from build123d import *

# Parameters (mm, degrees)
SKETCH1_W           = 254
SKETCH1_H           = 58.42
BOSS_EXTRUDE1_DEPTH = 19.05
CUT_EXTRUDE1_DEPTH  = 6.35
FILLET1_R           = 9.525
CUT_EXTRUDE2_START  = -127
SKETCH4_W           = 63.359739346
SKETCH4_H           = 23.579054397
CUT_EXTRUDE2_DEPTH  = 127
SKETCH5_R           = 3.175
CUT_EXTRUDE3_DEPTH  = 15.24
SKETCH6_W           = 12.7
SKETCH6_H           = 21.082
BOSS_EXTRUDE2_DEPTH = 6.35


with BuildPart() as part:
    # Sketch1 → Boss-Extrude1 (new body)
    with BuildSketch(Plane(origin=(0, 0, 0), x_dir=(1, 0, 0), z_dir=(0, 1, 0))):
        with Locations((127, 29.21)):
            Rectangle(SKETCH1_W, SKETCH1_H)
    extrude(amount=BOSS_EXTRUDE1_DEPTH)

    # Sketch2 → Cut-Extrude1 (cut)
    with BuildSketch(Plane(origin=(0, 19.05, 0), x_dir=(1, 0, 0), z_dir=(0, 1, 0))):
        Polygon((221.234, 52.07), (221.234, 18.288), (127, 18.288), (127, 0), (254, 0), (254, 58.42), (127, 58.42), (127, 52.07), align=None)
        Polygon((127, 0), (127, 18.288), (32.766, 18.288), (32.766, 52.07), (127, 52.07), (127, 58.42), (0, 58.42), (0, 0), align=None)
    extrude(amount=-CUT_EXTRUDE1_DEPTH, mode=Mode.SUBTRACT)

    # Fillet1
    fillet1_edges = [part.edges().sort_by_distance(p)[0] for p in [
        (254, 0, -29.21),
        (0, 0, -29.21),
    ]]
    fillet(fillet1_edges, radius=FILLET1_R)

    # Sketch4 → Cut-Extrude2 (cut)
    with BuildSketch(Plane(origin=(254, 0, 0), x_dir=(0, 0, -1), z_dir=(1, 0, 0)).offset(CUT_EXTRUDE2_START)):
        with Locations((31.679869673, 11.789527199)):
            Rectangle(SKETCH4_W, SKETCH4_H)
    extrude(amount=CUT_EXTRUDE2_DEPTH, mode=Mode.SUBTRACT)

    # Sketch5 → Cut-Extrude3 (cut)
    with BuildSketch(Plane(origin=(127, 0, 0), x_dir=(0, 0, -1), z_dir=(1, 0, 0))):
        with Locations((16.51, 6.35)):
            Circle(SKETCH5_R)
        with Locations((29.21, 6.35)):
            Circle(SKETCH5_R)
        with Locations((41.91, 6.35)):
            Circle(SKETCH5_R)
    extrude(amount=-CUT_EXTRUDE3_DEPTH, mode=Mode.SUBTRACT)

    # Sketch6 → Boss-Extrude2 (add)
    with BuildSketch(Plane(origin=(0, 12.7, 0), x_dir=(1, 0, 0), z_dir=(0, 1, 0))):
        with Locations((26.416, 28.829)):
            Rectangle(SKETCH6_W, SKETCH6_H)
    extrude(amount=BOSS_EXTRUDE2_DEPTH)


solid = part.part
Can you work these out from the model? Positions are in its coordinate system, mm. A direction names the side the tool comes from. Give positions to 0.01 mm unless a question says otherwise; leave off trailing zeros. Order: outer loops, then holes, each group sorted by start corner. A loop starts at its lowest first (then second) coordinate and runs counter-clockwise, first axis right, second up. Notation, with made-up numbers: M 88,19.5 L 139,19.5 A19 ccw 139,29.5 Z; hole C 72.25,-6.75 d5. An arc over 180 degrees is marked long. Use one line per item in the form item = value. Start each with the question number.
Item 1: Will these pins go through, and if not, where does the flat tip stop? pin 1 Ø7 at (x, y) = (25, 15.5) entering from -Z; pin 2 Ø4 at (y, z) = (6.35, -29.21) entering from +X; pin 3 Ø2 at (y, z) = (5.5, -6) entering from -X; pin 4 Ø1.5 at (y, z) = (16.5, -49.5) entering from -X.
Item 2: If we section it at B-B (x = 114): Write out the boundary of the cut face in (y, z) (3 decimals).
Item 3: We'd pull the mould along Y, two halves only. Please class faces 1 (the flat face through (73, 16, -18.288)), 2 (the flat face through (73, 19.05, -35)), 3 (the flat face through (111.76, 6, -42)), 4 (the cylindrical face through (2.72, 2.86, -29.62)): +Y half, -Y half, draft (parallel to the pull), parting line (faces both ways), or undercut.
Item 4: If we section it at D-D (z = -5.5): Write out the boundary of the cut face in (x, y) (3 decimals), then the cut area to 3 significant figures.
Item 5: For faces 5 (the flat face through (32.766, 16, -46)), 6 (the flat face through (20.066, 16, -29)), 7 (the cylindrical face through (119.5, 9.5, -16.1)), 8 (the flat face through (79, 16, -52.07)), which set-ups out of +Z, -Z, +X, -X, +Y, -Y let a thin tool reach every point of the face, with its end or its side?
Item 6: If we section it at C-C (y = 14.5): Write out the boundary of the cut face in (x, z).
Item 7: If I drill on line 1 along Y through (x, z) = (121, -29); line 2 along Y through (x, z) = (120.25, -16.51) (3 decimals); line 3 along Z through (x, y) = (50, 13.75), over which ranges is the centre line in solid material (lowest first)?
Item 8: If we section it at A-A (x = 29.5): Write out the boundary of the cut face in (y, z).
Outcome:
q1.pin_1 = -58.42
q1.pin_2 = 111.76
q1.pin_3 = 0.49
q1.pin_4 = 32.77
q2.outline = M 0,-58.42 L 12.7,-58.42 L 12.7,-52.07 L 19.05,-52.07 L 19.05,-18.288 L 12.7,-18.288 L 12.7,0 L 0,0 Z; hole C 6.35,-41.91 d6.35; hole C 6.35,-29.21 d6.35; hole C 6.35,-16.51 d6.35
q3.face_1 = draft
q3.face_2 = +Y half
q3.face_3 = undercut
q3.face_4 = -Y half
q4.outline = M 0,9.525 A9.525 ccw 9.525,0 L 127,0 L 127,12.7 L 0,12.7 Z
q4.area = 1,590 mm2
q5.face_5 = -Z, -X, +Y
q5.face_6 = +Z, -Z, -X, +Y
q5.face_7 = +X
q5.face_8 = -Z, +X, -X, +Y
q6.outline = M 20.07,-39.37 L 32.77,-39.37 L 32.77,-52.07 L 127,-52.07 L 127,-18.29 L 20.07,-18.29 Z
q7.line_1 = 0 to 3.18, 9.52 to 19.05
q7.line_2 = 0 to 3.175, 9.525 to 12.7
q7.line_3 = -52.07 to -18.29
q8.outline = M 0,-58.42 L 12.7,-58.42 L 12.7,-39.37 L 19.05,-39.37 L 19.05,-18.29 L 12.7,-18.29 L 12.7,0 L 0,0 Z
